Can you work these out from the model? Positions are in its coordinate system, mm. A direction names the side the tool comes from. Give positions to 0.01 mm unless a question says otherwise; leave off trailing zeros. Write each loop counter-clockwise with the first axis right and the second up, starting at its lowest first coordinate (ties: lowest second). Pieces come first, ordered by that corner, then holes.
```python
from build123d import *

# Parameters (mm, degrees)
F0_R     = 20
F0_R_2   = 16
F0_R_3   = 14
F0_R_4   = 12
F1_DEPTH = 20
F2_DEPTH = 16
F3_DEPTH = 6
F4_DEPTH = 3.5


with BuildPart() as f1:
    # F0 (on Top) → F1 (new body)
    with BuildSketch(Plane.XY):
        Circle(F0_R)
        Circle(F0_R_2, mode=Mode.SUBTRACT)
        Circle(F0_R_2)
        Circle(F0_R_3, mode=Mode.SUBTRACT)
        Circle(F0_R_3)
        Circle(F0_R_4, mode=Mode.SUBTRACT)
        Circle(F0_R_4)
    extrude(amount=-F1_DEPTH)

    # F0 (on Top) → F2 (cut)
    with BuildSketch(Plane.XY):
        Circle(F0_R_4)
    extrude(amount=-F2_DEPTH, mode=Mode.SUBTRACT)

    # F0 (on Top) → F3 (cut)
    with BuildSketch(Plane.XY):
        Circle(F0_R_3)
        Circle(F0_R_4, mode=Mode.SUBTRACT)
    extrude(amount=-F3_DEPTH, mode=Mode.SUBTRACT)

    # F0 (on Top) → F4 (cut)
    with BuildSketch(Plane.XY):
        Circle(F0_R_2)
        Circle(F0_R_3, mode=Mode.SUBTRACT)
    extrude(amount=-F4_DEPTH, mode=Mode.SUBTRACT)


solid = f1.part
```
1) If we mould it in two halves opening along X, with no side actions, what happens to faces 3 (the face through (-6.3, 10.4, -6)), 4 (the face through (-4.336, -19.524, -9.86)), 5 (the face through (-11.99, 0.53, -10.93)), 6 (the face through (-8.98, 13.43, 0))? For each: +X half, -X half, draft (parallel to the pull), parting line (faces both ways), or undercut.
Values follow:
face 3: undercut
face 4: parting line
face 5: undercut
face 6: draft
2) For faces 1 (the face through (-3.47, -15.62, -1.73)), 2 (the face through (0, 0, -20)), which set-ups out of +Z, -Z, +X, -X, +Y, -Y let a thin tool reach every point of the face, with its end or its side?
Values follow:
face 1: +Z
face 2: -Z, +X, -X, +Y, -Y
3) Please list where these lines run through material, in increasing order: L1, parallel to Y at x = 0, z = -9; L2, parallel to Y at x = 0, z = -1.35; L3, parallel to Z at x = -3, y = 9.
Values follow:
L1: y = -20 to -12, 12 to 20
L2: y = -20 to -16, 16 to 20
L3: z = -20 to -16
4) Suppose I cut it at B-B on z = -11.5. Write out the boundary of the cut face in (x, y).
Values follow:
outline: circle Ø40 at (0, 0); hole circle Ø24 at (0, 0)
5) Suppose I cut it at D-D on z = -17. Write out the boundary of the cut face in (x, y).
Values follow:
outline: circle Ø40 at (0, 0)
6) Suppose I cut it at A-A on x = 0. Write out the boundary of the cut face in (y, z), plus the area to 3 significant figures.
Values follow:
outline: (-20, -20) - (20, -20) - (20, 0) - (16, 0) - (16, -3.5) - (14, -3.5) - (14, -6) - (12, -6) - (12, -16) - (-12, -16) - (-12, -6) - (-14, -6) - (-14, -3.5) - (-16, -3.5) - (-16, 0) - (-20, 0) - close
area: 378 mm2
7) For pin 1 Ø3 at (x, y) = (-11, 0.5) entering from +Z; pin 2 Ø1 at (y, z) = (-2, -7.5) entering from -X; pin 3 Ø8 at (y, z) = (-10.5, -9.5) entering from -X, each with a flat end and sliding along its axis, tell me the tip position at first contact or that it passes through.
Values follow:
pin 1: stops at z = -6
pin 2: stops at x = -19.94
pin 3: stops at x = -18.91
